Verification items for the finished model (mm, model axes). Give positions to 0.01 mm unless a question says otherwise; leave off trailing zeros. Order: outer loops, then holes, each group sorted by start corner. A loop starts at its lowest first (then second) coordinate and runs counter-clockwise, first axis right, second up. Notation, with made-up numbers: (-6.75, -36.75) -> (28.25, -36.75) arc R10 ccw to (28.25, -26.75) -> close; hole circle Ø6 at (38.25, -3.75). An arc over 180 degrees is marked (long way). Write each question's results on one line, items separated by ' | '. Start each with the question number.
1. Cross-section at A-A, the plane z = -8.5. Enter the section's corners in (x, y), then the cut area to 3 significant figures.
2. Cross-section at B-B, the plane x = -57.5. Enter the section's corners in (y, z).
3. Mould release check, pull along X, two halves, no side actions. Record for faces 1 (the face through (58, 2, -74)), 2 (the face through (-55.974, 1.972, -51.981)), 3 (the face through (-59, 2, -73)), 4 (the face through (-1, 2, 75)): +X half, -X half, draft (parallel to the pull), parting line (faces both ways), or undercut.
4. Material ranges on L1, parallel to Z at x = -37.75, y = 2.85; L2, parallel to X at y = 2.5, z = -51.5; L3, parallel to X at y = 2.05, z = 18.6, recorded low to high. Write a range as from..to.
from build123d import *

# Parameters (mm, degrees)
SKETCH_1_W      = 120
SKETCH_1_H      = 150
SKETCH_1_R      = 1.6
SKETCH_1_R_2    = 1.1
EXTRUDE_1_DEPTH = 4
FILLET_1_R      = 5


with BuildPart() as part:
    # 草图1 → 凸台-拉伸1 (new body)
    with BuildSketch(Plane(origin=(0, 0, 0), x_dir=(1, 0, 0), z_dir=(0, 1, 0))):
        Rectangle(SKETCH_1_W, SKETCH_1_H)
        with Locations((-57.5, 51.5)):
            Circle(SKETCH_1_R, mode=Mode.SUBTRACT)
        with Locations((-57.5, 8.5)):
            Circle(SKETCH_1_R, mode=Mode.SUBTRACT)
        with Locations((-37.75, 35.23)):
            Circle(SKETCH_1_R, mode=Mode.SUBTRACT)
        with Locations((-37.75, 24.77)):
            Circle(SKETCH_1_R, mode=Mode.SUBTRACT)
        with Locations((-57.5, -8.5)):
            Circle(SKETCH_1_R, mode=Mode.SUBTRACT)
        with Locations((-37.75, -24.77)):
            Circle(SKETCH_1_R, mode=Mode.SUBTRACT)
        with Locations((-37.75, -35.23)):
            Circle(SKETCH_1_R, mode=Mode.SUBTRACT)
        with Locations((-57.5, -51.5)):
            Circle(SKETCH_1_R, mode=Mode.SUBTRACT)
        with Locations((57.5, -51.5)):
            Circle(SKETCH_1_R, mode=Mode.SUBTRACT)
        with Locations((37.75, -35.23)):
            Circle(SKETCH_1_R, mode=Mode.SUBTRACT)
        with Locations((37.75, -24.77)):
            Circle(SKETCH_1_R, mode=Mode.SUBTRACT)
        with Locations((57.5, -8.5)):
            Circle(SKETCH_1_R, mode=Mode.SUBTRACT)
        with Locations((57.5, 8.5)):
            Circle(SKETCH_1_R, mode=Mode.SUBTRACT)
        with Locations((37.75, 24.77)):
            Circle(SKETCH_1_R, mode=Mode.SUBTRACT)
        with Locations((37.75, 35.23)):
            Circle(SKETCH_1_R, mode=Mode.SUBTRACT)
        with Locations((57.5, 51.5)):
            Circle(SKETCH_1_R, mode=Mode.SUBTRACT)
        with Locations((0, 18.6)):
            Circle(SKETCH_1_R_2, mode=Mode.SUBTRACT)
        with Locations((8.8, -18.6)):
            Circle(SKETCH_1_R_2, mode=Mode.SUBTRACT)
        with Locations((-8.8, -18.6)):
            Circle(SKETCH_1_R_2, mode=Mode.SUBTRACT)
        with Locations((-21, 25)):
            Circle(SKETCH_1_R, mode=Mode.SUBTRACT)
        with Locations((21, 25)):
            Circle(SKETCH_1_R, mode=Mode.SUBTRACT)
        with Locations((21, -25)):
            Circle(SKETCH_1_R, mode=Mode.SUBTRACT)
        with Locations((-21, -25)):
            Circle(SKETCH_1_R, mode=Mode.SUBTRACT)
    extrude(amount=EXTRUDE_1_DEPTH)

    # 圆角1
    fillet_1_edges = [part.edges().sort_by_distance(p)[0] for p in [
        (60, 2, 75),
        (-60, 2, 75),
        (-60, 2, -75),
        (60, 2, -75),
    ]]
    fillet(fillet_1_edges, radius=FILLET_1_R)


solid = part.part
Results below:
1) outline: (-60, 0) -> (-59.1, 0) -> (-59.1, 4) -> (-60, 4) -> close; (-55.9, 0) -> (55.9, 0) -> (55.9, 4) -> (-55.9, 4) -> close; (59.1, 0) -> (60, 0) -> (60, 4) -> (59.1, 4) -> close | area: 454 mm²
2) outline: (0, -74.33) -> (4, -74.33) -> (4, -53.1) -> (0, -53.1) -> close; (0, -49.9) -> (4, -49.9) -> (4, -10.1) -> (0, -10.1) -> close; (0, -6.9) -> (4, -6.9) -> (4, 6.9) -> (0, 6.9) -> close; (0, 10.1) -> (4, 10.1) -> (4, 49.9) -> (0, 49.9) -> close; (0, 53.1) -> (4, 53.1) -> (4, 74.33) -> (0, 74.33) -> close
3) face 1: +X half | face 2: undercut | face 3: -X half | face 4: draft
4) L1: z = -75..-36.83, -33.63..-26.37, -23.17..23.17, 26.37..33.63, 36.83..75 | L2: x = -60..-59.1, -55.9..55.9, 59.1..60 | L3: x = -60..-9.9, -7.7..7.7, 9.9..60
